Check sheet for the modelled part. Datum: model origin and axes. Units: mm. Coordinates: 2 decimals unless noted, no trailing zeros.
1. Thickness scan on line 1 (Y direction, x = 20, z = 5.25); line 2 (X direction, y = 75.5, z = 8); line 3 (Y direction, x = 120, z = 7.75). Record the ranges inside material, lowest first.
2. Cross-section at A-A (z = 5.75). Count the separate pieces of the cut face and the enclosed holes in it, then the cut area to 3 significant figures.
3. Gauge pin test, flat ends, axial feed: pin 1 Ø3 at (x, y) = (120, 90) entering from +Z; pin 2 Ø3.5 at (x, y) = (80, 16.81) entering from -Z; pin 3 Ø2.5 at (x, y) = (19, 17.5) entering from -Z. Record the tip position at first contact, or that the pin passes through.
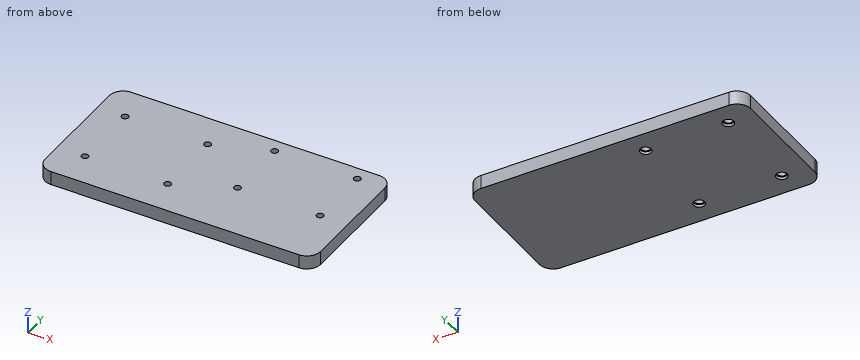
```python
from build123d import *

# Parameters (mm, degrees)
SKETCH4_W                                     = 200
SKETCH4_H                                     = 100
BOSS_EXTRUDE1_DEPTH                           = 10
CBORE_FOR_M6_HEX_HEAD_CAP_SCREW7_D            = 6
CBORE_FOR_M6_HEX_HEAD_CAP_SCREW7_DEPTH        = 8
CBORE_FOR_M6_HEX_HEAD_CAP_SCREW7_CBORE_D      = 8
CBORE_FOR_M6_HEX_HEAD_CAP_SCREW7_CBORE_DEPTH  = 2
CBORE_FOR_M6_HEX_HEAD_CAP_SCREW7_TIP          = 1.802581857
CBORE_FOR_M6_HEX_HEAD_CAP_SCREW8_D            = 6
CBORE_FOR_M6_HEX_HEAD_CAP_SCREW8_DEPTH        = 8
CBORE_FOR_M6_HEX_HEAD_CAP_SCREW8_CBORE_D      = 8
CBORE_FOR_M6_HEX_HEAD_CAP_SCREW8_CBORE_DEPTH  = 2
CBORE_FOR_M6_HEX_HEAD_CAP_SCREW8_TIP          = 1.802581857
CBORE_FOR_M6_HEX_HEAD_CAP_SCREW9_D            = 6
CBORE_FOR_M6_HEX_HEAD_CAP_SCREW9_DEPTH        = 8
CBORE_FOR_M6_HEX_HEAD_CAP_SCREW9_CBORE_D      = 8
CBORE_FOR_M6_HEX_HEAD_CAP_SCREW9_CBORE_DEPTH  = 2
CBORE_FOR_M6_HEX_HEAD_CAP_SCREW9_TIP          = 1.802581857
CBORE_FOR_M6_HEX_HEAD_CAP_SCREW10_D           = 6
CBORE_FOR_M6_HEX_HEAD_CAP_SCREW10_DEPTH       = 8
CBORE_FOR_M6_HEX_HEAD_CAP_SCREW10_CBORE_D     = 8
CBORE_FOR_M6_HEX_HEAD_CAP_SCREW10_CBORE_DEPTH = 2
CBORE_FOR_M6_HEX_HEAD_CAP_SCREW10_TIP         = 1.802581857
F_1_0_1_DIAMETER_HOLE7_D                      = 5
F_1_0_1_DIAMETER_HOLE7_DEPTH                  = 8
F_1_0_1_DIAMETER_HOLE7_TIP                    = 1.502151548
F_1_0_1_DIAMETER_HOLE8_D                      = 5
F_1_0_1_DIAMETER_HOLE8_DEPTH                  = 8
F_1_0_1_DIAMETER_HOLE8_TIP                    = 1.502151548
F_1_0_1_DIAMETER_HOLE9_D                      = 5
F_1_0_1_DIAMETER_HOLE9_DEPTH                  = 8
F_1_0_1_DIAMETER_HOLE9_TIP                    = 1.502151548
F_1_0_1_DIAMETER_HOLE10_D                     = 5
F_1_0_1_DIAMETER_HOLE10_DEPTH                 = 8
F_1_0_1_DIAMETER_HOLE10_TIP                   = 1.502151548
F_5_0_5_DIAMETER_HOLE1_D                      = 5
F_5_0_5_DIAMETER_HOLE1_DEPTH                  = 8
F_5_0_5_DIAMETER_HOLE1_TIP                    = 1.502151548
F_5_0_5_DIAMETER_HOLE2_D                      = 5
F_5_0_5_DIAMETER_HOLE2_DEPTH                  = 8
F_5_0_5_DIAMETER_HOLE2_TIP                    = 1.502151548
F_5_0_5_DIAMETER_HOLE3_D                      = 5
F_5_0_5_DIAMETER_HOLE3_DEPTH                  = 8
F_5_0_5_DIAMETER_HOLE3_TIP                    = 1.502151548
F_5_0_5_DIAMETER_HOLE5_D                      = 5
F_5_0_5_DIAMETER_HOLE5_DEPTH                  = 8
F_5_0_5_DIAMETER_HOLE5_TIP                    = 1.502151548
FILLET1_R                                     = 10
FILLET2_R                                     = 10
FILLET3_R                                     = 10
FILLET4_R                                     = 10
CBORE_FOR_M6_HEX_HEAD_CAP_SCREW3_D            = 6
CBORE_FOR_M6_HEX_HEAD_CAP_SCREW3_DEPTH        = 8
CBORE_FOR_M6_HEX_HEAD_CAP_SCREW3_CBORE_D      = 8
CBORE_FOR_M6_HEX_HEAD_CAP_SCREW3_CBORE_DEPTH  = 2
CBORE_FOR_M6_HEX_HEAD_CAP_SCREW3_TIP          = 1.802581857
CBORE_FOR_M6_HEX_HEAD_CAP_SCREW4_D            = 6
CBORE_FOR_M6_HEX_HEAD_CAP_SCREW4_DEPTH        = 8
CBORE_FOR_M6_HEX_HEAD_CAP_SCREW4_CBORE_D      = 8
CBORE_FOR_M6_HEX_HEAD_CAP_SCREW4_CBORE_DEPTH  = 2
CBORE_FOR_M6_HEX_HEAD_CAP_SCREW4_TIP          = 1.802581857
CBORE_FOR_M6_HEX_HEAD_CAP_SCREW6_D            = 6
CBORE_FOR_M6_HEX_HEAD_CAP_SCREW6_DEPTH        = 8
CBORE_FOR_M6_HEX_HEAD_CAP_SCREW6_CBORE_D      = 8
CBORE_FOR_M6_HEX_HEAD_CAP_SCREW6_CBORE_DEPTH  = 2
CBORE_FOR_M6_HEX_HEAD_CAP_SCREW6_TIP          = 1.802581857


with BuildPart() as part:
    # Sketch4 → Boss-Extrude1 (new body)
    with BuildSketch(Plane.XY):
        with Locations((100, 50)):
            Rectangle(SKETCH4_W, SKETCH4_H)
    extrude(amount=BOSS_EXTRUDE1_DEPTH)

    # CBORE for M6 Hex Head Cap Screw7
    with Locations(Plane(origin=(0, 0, 0), x_dir=(-1, 0, 0), z_dir=(0, 0, -1))):
        with Locations((-80, 83.464013217)):
            CounterBoreHole(CBORE_FOR_M6_HEX_HEAD_CAP_SCREW7_D / 2, CBORE_FOR_M6_HEX_HEAD_CAP_SCREW7_CBORE_D / 2, CBORE_FOR_M6_HEX_HEAD_CAP_SCREW7_CBORE_DEPTH, depth=CBORE_FOR_M6_HEX_HEAD_CAP_SCREW7_DEPTH)
            with Locations((0, 0, -(CBORE_FOR_M6_HEX_HEAD_CAP_SCREW7_DEPTH + CBORE_FOR_M6_HEX_HEAD_CAP_SCREW7_TIP / 2))):  # 118° drill point
                Cone(0, CBORE_FOR_M6_HEX_HEAD_CAP_SCREW7_D / 2, CBORE_FOR_M6_HEX_HEAD_CAP_SCREW7_TIP, mode=Mode.SUBTRACT)

    # CBORE for M6 Hex Head Cap Screw8
    with Locations(Plane(origin=(0, 0, 0), x_dir=(-1, 0, 0), z_dir=(0, 0, -1))):
        with Locations((-20, 83.464013217)):
            CounterBoreHole(CBORE_FOR_M6_HEX_HEAD_CAP_SCREW8_D / 2, CBORE_FOR_M6_HEX_HEAD_CAP_SCREW8_CBORE_D / 2, CBORE_FOR_M6_HEX_HEAD_CAP_SCREW8_CBORE_DEPTH, depth=CBORE_FOR_M6_HEX_HEAD_CAP_SCREW8_DEPTH)
            with Locations((0, 0, -(CBORE_FOR_M6_HEX_HEAD_CAP_SCREW8_DEPTH + CBORE_FOR_M6_HEX_HEAD_CAP_SCREW8_TIP / 2))):  # 118° drill point
                Cone(0, CBORE_FOR_M6_HEX_HEAD_CAP_SCREW8_D / 2, CBORE_FOR_M6_HEX_HEAD_CAP_SCREW8_TIP, mode=Mode.SUBTRACT)

    # CBORE for M6 Hex Head Cap Screw9
    with Locations(Plane(origin=(0, 0, 0), x_dir=(-1, 0, 0), z_dir=(0, 0, -1))):
        with Locations((-20, 16.814013217)):
            CounterBoreHole(CBORE_FOR_M6_HEX_HEAD_CAP_SCREW9_D / 2, CBORE_FOR_M6_HEX_HEAD_CAP_SCREW9_CBORE_D / 2, CBORE_FOR_M6_HEX_HEAD_CAP_SCREW9_CBORE_DEPTH, depth=CBORE_FOR_M6_HEX_HEAD_CAP_SCREW9_DEPTH)
            with Locations((0, 0, -(CBORE_FOR_M6_HEX_HEAD_CAP_SCREW9_DEPTH + CBORE_FOR_M6_HEX_HEAD_CAP_SCREW9_TIP / 2))):  # 118° drill point
                Cone(0, CBORE_FOR_M6_HEX_HEAD_CAP_SCREW9_D / 2, CBORE_FOR_M6_HEX_HEAD_CAP_SCREW9_TIP, mode=Mode.SUBTRACT)

    # CBORE for M6 Hex Head Cap Screw10
    with Locations(Plane(origin=(0, 0, 0), x_dir=(-1, 0, 0), z_dir=(0, 0, -1))):
        with Locations((-80, 16.814013217)):
            CounterBoreHole(CBORE_FOR_M6_HEX_HEAD_CAP_SCREW10_D / 2, CBORE_FOR_M6_HEX_HEAD_CAP_SCREW10_CBORE_D / 2, CBORE_FOR_M6_HEX_HEAD_CAP_SCREW10_CBORE_DEPTH, depth=CBORE_FOR_M6_HEX_HEAD_CAP_SCREW10_DEPTH)
            with Locations((0, 0, -(CBORE_FOR_M6_HEX_HEAD_CAP_SCREW10_DEPTH + CBORE_FOR_M6_HEX_HEAD_CAP_SCREW10_TIP / 2))):  # 118° drill point
                Cone(0, CBORE_FOR_M6_HEX_HEAD_CAP_SCREW10_D / 2, CBORE_FOR_M6_HEX_HEAD_CAP_SCREW10_TIP, mode=Mode.SUBTRACT)

    # Ø1.0 (1) Diameter Hole7
    with Locations(Plane.XY.offset(10)):
        with Locations((20, 75.196019825)):
            Hole(F_1_0_1_DIAMETER_HOLE7_D / 2, depth=F_1_0_1_DIAMETER_HOLE7_DEPTH)
            with Locations((0, 0, -(F_1_0_1_DIAMETER_HOLE7_DEPTH + F_1_0_1_DIAMETER_HOLE7_TIP / 2))):  # 118° drill point
                Cone(0, F_1_0_1_DIAMETER_HOLE7_D / 2, F_1_0_1_DIAMETER_HOLE7_TIP, mode=Mode.SUBTRACT)

    # Ø1.0 (1) Diameter Hole8
    with Locations(Plane.XY.offset(10)):
        with Locations((80, 75.196019825)):
            Hole(F_1_0_1_DIAMETER_HOLE8_D / 2, depth=F_1_0_1_DIAMETER_HOLE8_DEPTH)
            with Locations((0, 0, -(F_1_0_1_DIAMETER_HOLE8_DEPTH + F_1_0_1_DIAMETER_HOLE8_TIP / 2))):  # 118° drill point
                Cone(0, F_1_0_1_DIAMETER_HOLE8_D / 2, F_1_0_1_DIAMETER_HOLE8_TIP, mode=Mode.SUBTRACT)

    # Ø1.0 (1) Diameter Hole9
    with Locations(Plane.XY.offset(10)):
        with Locations((20, 25.221019825)):
            Hole(F_1_0_1_DIAMETER_HOLE9_D / 2, depth=F_1_0_1_DIAMETER_HOLE9_DEPTH)
            with Locations((0, 0, -(F_1_0_1_DIAMETER_HOLE9_DEPTH + F_1_0_1_DIAMETER_HOLE9_TIP / 2))):  # 118° drill point
                Cone(0, F_1_0_1_DIAMETER_HOLE9_D / 2, F_1_0_1_DIAMETER_HOLE9_TIP, mode=Mode.SUBTRACT)

    # Ø1.0 (1) Diameter Hole10
    with Locations(Plane.XY.offset(10)):
        with Locations((80, 25.221019825)):
            Hole(F_1_0_1_DIAMETER_HOLE10_D / 2, depth=F_1_0_1_DIAMETER_HOLE10_DEPTH)
            with Locations((0, 0, -(F_1_0_1_DIAMETER_HOLE10_DEPTH + F_1_0_1_DIAMETER_HOLE10_TIP / 2))):  # 118° drill point
                Cone(0, F_1_0_1_DIAMETER_HOLE10_D / 2, F_1_0_1_DIAMETER_HOLE10_TIP, mode=Mode.SUBTRACT)

    # Ø5.0 (5) Diameter Hole1
    with Locations(Plane.XY.offset(10)):
        with Locations((120, 90)):
            Hole(F_5_0_5_DIAMETER_HOLE1_D / 2, depth=F_5_0_5_DIAMETER_HOLE1_DEPTH)
            with Locations((0, 0, -(F_5_0_5_DIAMETER_HOLE1_DEPTH + F_5_0_5_DIAMETER_HOLE1_TIP / 2))):  # 118° drill point
                Cone(0, F_5_0_5_DIAMETER_HOLE1_D / 2, F_5_0_5_DIAMETER_HOLE1_TIP, mode=Mode.SUBTRACT)

    # Ø5.0 (5) Diameter Hole2
    with Locations(Plane.XY.offset(10)):
        with Locations((180, 90)):
            Hole(F_5_0_5_DIAMETER_HOLE2_D / 2, depth=F_5_0_5_DIAMETER_HOLE2_DEPTH)
            with Locations((0, 0, -(F_5_0_5_DIAMETER_HOLE2_DEPTH + F_5_0_5_DIAMETER_HOLE2_TIP / 2))):  # 118° drill point
                Cone(0, F_5_0_5_DIAMETER_HOLE2_D / 2, F_5_0_5_DIAMETER_HOLE2_TIP, mode=Mode.SUBTRACT)

    # Ø5.0 (5) Diameter Hole3
    with Locations(Plane.XY.offset(10)):
        with Locations((120, 43.628026433)):
            Hole(F_5_0_5_DIAMETER_HOLE3_D / 2, depth=F_5_0_5_DIAMETER_HOLE3_DEPTH)
            with Locations((0, 0, -(F_5_0_5_DIAMETER_HOLE3_DEPTH + F_5_0_5_DIAMETER_HOLE3_TIP / 2))):  # 118° drill point
                Cone(0, F_5_0_5_DIAMETER_HOLE3_D / 2, F_5_0_5_DIAMETER_HOLE3_TIP, mode=Mode.SUBTRACT)

    # Ø5.0 (5) Diameter Hole5
    with Locations(Plane.XY.offset(10)):
        with Locations((180, 43.628026433)):
            Hole(F_5_0_5_DIAMETER_HOLE5_D / 2, depth=F_5_0_5_DIAMETER_HOLE5_DEPTH)
            with Locations((0, 0, -(F_5_0_5_DIAMETER_HOLE5_DEPTH + F_5_0_5_DIAMETER_HOLE5_TIP / 2))):  # 118° drill point
                Cone(0, F_5_0_5_DIAMETER_HOLE5_D / 2, F_5_0_5_DIAMETER_HOLE5_TIP, mode=Mode.SUBTRACT)

    # Fillet1
    fillet1_edges = [part.edges().sort_by_distance(p)[0] for p in [
        (0, 100, 5),
    ]]
    fillet(fillet1_edges, radius=FILLET1_R)

    # Fillet2
    fillet2_edges = [part.edges().sort_by_distance(p)[0] for p in [
        (0, 0, 5),
    ]]
    fillet(fillet2_edges, radius=FILLET2_R)

    # Fillet3
    fillet3_edges = [part.edges().sort_by_distance(p)[0] for p in [
        (200, 0, 5),
    ]]
    fillet(fillet3_edges, radius=FILLET3_R)

    # Fillet4
    fillet4_edges = [part.edges().sort_by_distance(p)[0] for p in [
        (200, 100, 5),
    ]]
    fillet(fillet4_edges, radius=FILLET4_R)

    # CBORE for M6 Hex Head Cap Screw3
    with Locations(Plane(origin=(0, 0, 0), x_dir=(-1, 0, 0), z_dir=(0, 0, -1))):
        with Locations((-80, 16.814013217)):
            CounterBoreHole(CBORE_FOR_M6_HEX_HEAD_CAP_SCREW3_D / 2, CBORE_FOR_M6_HEX_HEAD_CAP_SCREW3_CBORE_D / 2, CBORE_FOR_M6_HEX_HEAD_CAP_SCREW3_CBORE_DEPTH, depth=CBORE_FOR_M6_HEX_HEAD_CAP_SCREW3_DEPTH)
            with Locations((0, 0, -(CBORE_FOR_M6_HEX_HEAD_CAP_SCREW3_DEPTH + CBORE_FOR_M6_HEX_HEAD_CAP_SCREW3_TIP / 2))):  # 118° drill point
                Cone(0, CBORE_FOR_M6_HEX_HEAD_CAP_SCREW3_D / 2, CBORE_FOR_M6_HEX_HEAD_CAP_SCREW3_TIP, mode=Mode.SUBTRACT)

    # CBORE for M6 Hex Head Cap Screw4
    with Locations(Plane(origin=(0, 0, 0), x_dir=(-1, 0, 0), z_dir=(0, 0, -1))):
        with Locations((-20, 16.814013217)):
            CounterBoreHole(CBORE_FOR_M6_HEX_HEAD_CAP_SCREW4_D / 2, CBORE_FOR_M6_HEX_HEAD_CAP_SCREW4_CBORE_D / 2, CBORE_FOR_M6_HEX_HEAD_CAP_SCREW4_CBORE_DEPTH, depth=CBORE_FOR_M6_HEX_HEAD_CAP_SCREW4_DEPTH)
            with Locations((0, 0, -(CBORE_FOR_M6_HEX_HEAD_CAP_SCREW4_DEPTH + CBORE_FOR_M6_HEX_HEAD_CAP_SCREW4_TIP / 2))):  # 118° drill point
                Cone(0, CBORE_FOR_M6_HEX_HEAD_CAP_SCREW4_D / 2, CBORE_FOR_M6_HEX_HEAD_CAP_SCREW4_TIP, mode=Mode.SUBTRACT)

    # CBORE for M6 Hex Head Cap Screw6
    with Locations(Plane(origin=(0, 0, 0), x_dir=(-1, 0, 0), z_dir=(0, 0, -1))):
        with Locations((-20, 83.464013217)):
            CounterBoreHole(CBORE_FOR_M6_HEX_HEAD_CAP_SCREW6_D / 2, CBORE_FOR_M6_HEX_HEAD_CAP_SCREW6_CBORE_D / 2, CBORE_FOR_M6_HEX_HEAD_CAP_SCREW6_CBORE_DEPTH, depth=CBORE_FOR_M6_HEX_HEAD_CAP_SCREW6_DEPTH)
            with Locations((0, 0, -(CBORE_FOR_M6_HEX_HEAD_CAP_SCREW6_DEPTH + CBORE_FOR_M6_HEX_HEAD_CAP_SCREW6_TIP / 2))):  # 118° drill point
                Cone(0, CBORE_FOR_M6_HEX_HEAD_CAP_SCREW6_D / 2, CBORE_FOR_M6_HEX_HEAD_CAP_SCREW6_TIP, mode=Mode.SUBTRACT)


solid = part.part
```
Data:
1. line 1: y = 0 to 13.81, 19.81 to 22.72, 27.72 to 72.7, 77.7 to 80.46, 86.46 to 100
1. line 2: x = 0 to 17.52, 22.48 to 77.52, 82.48 to 200
1. line 3: y = 0 to 41.13, 46.13 to 87.5, 92.5 to 100
2. separate pieces: 1
2. enclosed holes: 12
2. area: 19,600 mm2
3. pin 1: stops at z = 1.4
3. pin 2: stops at z = 8.75
3. pin 3: stops at z = 8.32
